For this review, take the finished solid that the model builds, in its own axes (mm). Face numbers are marked on the shaded views. A direction names the side the tool comes from. Round coordinates to 2 decimals unless told otherwise and drop trailing zeros. Loops run counter-clockwise (first coordinate to the right, second up) from the corner with the lowest first, then second, coordinate; pieces in that order, holes last.
1) Take a section at A-A (y = 2.25). State the section outline as (x, z) points.
2) Take a section at C-C (z = 1.75). State the section outline as (x, y) points, then the cut area to 3 significant figures.
3) Tool access review of the marked faces 4 and 5: name each direction out of +Z, -Z, +X, -X, +Y, -Y from which nothing blocks a thin tool from reaching the whole face with its end or side.
4) Wall thickness on L1, parallel to Z at x = -3.5, y = 5.25; L2, parallel to Y at x = 0.25, z = 1; L3, parallel to Y at x = 1.75, z = 1.5: over which ranges is each line inside the solid? List them lowest first.
5) Insertion check: pin 1 (1.5 mm diameter, centred on y = 5, z = 2, fed in from +X); pin 2 (1 mm diameter, centred on y = 6, z = 5, fed in from +X). Each pin has a flat end and moves straight along its axis. Give the tip position at first contact, or say it passes through.
6) Take a section at D-D (y = 1). State the section outline as (x, z) points, then the cut area to 3 significant figures.
7) Take a section at B-B (x = 2). State the section outline as (y, z) points.
8) Mouldability with a two-part tool opening along Z and no side actions: class the marked faces 1, 2 and 3 as pulls with the +Z half, pulls with the -Z half, needs draft (parallel to the pull), parting line crosses it, or undercut.
Autodesk Inventor part; units mm, degrees
ref_plane "作業平面1" through (-1.8159, 9, 6.1283) normal (0, 0.2337903, -0.972287) x (1, 0, 0)
ref_plane "YZ Plane" through (0, 0, 0) normal (1, 0, 0) x (0, 1, 0)
ref_plane "XZ Plane" through (0, 0, 0) normal (0, 1, 0) x (-1, 0, 0)
sketch "スケッチ1" plane through (0, 0, 0) normal (0, 0, 1) x (1, 0, 0)
  line L0 (-5, 9) -> (5, 9)
  line L1 (5, 9) -> (5, 0)
  line L2 (5, 0) -> (-5, 0)
  line L3 (-5, 0) -> (-5, 9)
  line L4 (-8.0749, 9) -> (-5, 9) construction
  point P0 (0, 0)
  point P1 (0, 9)
  point P2 (0, 0)
  dimension "d0" = 9
  dimension "d1" = 10
  dimension "d2" = 10
extrude "押し出し1" add sketch "スケッチ1" along normal blind 3
sketch "スケッチ2" plane through (-5, 9, 0) normal (0, 1, 0) x (1, 0, 0)
  line L0 (0, -3) -> (10, -3)
  line L1 (0, 0) -> (10, 0)
  line L2 (2.5173, -3) -> (0, 0)
  line L3 (10, 0) -> (7.4827, -3)
  line L4 (0, 0) -> (0, -3)
  line L5 (10, 0) -> (10, -3)
  point P0 (5, 0)
  dimension "d5" = 80
  dimension "d6" = 40
  dimension "d7" = 40
extrude "押し出し2" cut sketch "スケッチ2" against normal through all contours L4 L2 L0 | L3 L5 L0
sketch "スケッチ3" plane through (-5, 0, 0) normal (-0.7660444, 0, 0.6427876) x (0.6427876, 0, 0.7660444)
  line L0 (3.9162, 0) -> (0, 0)
  line L1 (3.9162, 9) -> (3.9162, 0)
  line L2 (0, 9) -> (3.9162, 9)
  line L3 (0, 9) -> (0, 0)
  line L4 (3.9162, 0) -> (7.1079, 0)
  line L5 (3.9162, 0) -> (-11.0838, 7)
  point P0 (3.2139, 0)
  point P1 (0, 1.8276)
  dimension "d10" = 15
  dimension "d11" = 7
extrude "押し出し3" cut sketch "スケッチ3" against normal through all contours L0 L3 L5
sketch "スケッチ4" plane through (5, 0, 0) normal (0.7660444, 0, 0.6427876) x (0.6427876, 0, -0.7660444)
  line L0 (0, 0) -> (-3.9162, 0)
  line L1 (0, 0) -> (0, 9)
  line L2 (-3.9162, 9) -> (0, 9)
  line L3 (-3.9162, 0) -> (-3.9162, 9)
  line L4 (-3.9162, 0) -> (11.0838, 7)
  point P0 (-3.2139, 0)
  point P1 (0, 1.8276)
  dimension "d14" = 15
  dimension "d15" = 7
extrude "押し出し4" cut sketch "スケッチ4" against normal through all contours L0 L4 L1
sketch "スケッチ5" plane through (0, 0, 3) normal (0, 0, 1) x (1, 0, 0)
  line L0 (-2.4827, 9) -> (-2.4827, 0)
  line L1 (-2.4827, 0) -> (2.4827, 0)
  line L2 (2.4827, 0) -> (2.4827, 9)
  line L3 (2.4827, 9) -> (-2.4827, 9)
  point P0 (0, 0)
extrude "押し出し5" add sketch "スケッチ5" along normal blind 10
sketch "スケッチ6" plane through (-2.4827, 0, 3) normal (-1, 0, 0) x (0, 0, 1)
  line L0 (0, 9) -> (0, 0)
  line L1 (0, 0) -> (10, 0)
  line L2 (10, 9) -> (10, 0)
  line L3 (0, 9) -> (10, 9)
  point P0 (-3, 0)
extrude "押し出し6" add sketch "スケッチ6" along normal blind 10
sketch "スケッチ7" plane through (2.4827, 0, 3) normal (1, 0, 0) x (0, 0, -1)
  line L0 (0, 0) -> (0, 9)
  line L1 (0, 9) -> (-10, 9)
  line L2 (-10, 0) -> (-10, 9)
  line L3 (0, 0) -> (-10, 0)
  point P0 (3, 0)
extrude "押し出し7" add sketch "スケッチ7" along normal blind 10
sketch "スケッチ8" plane through (5, 1.8276, 0) normal (0.7660444, 0, 0.6427876) x (0.6427876, 0, -0.7660444)
  line L0 (-7.1079, 7.1724) -> (-7.1079, -1.8276)
  line L1 (-3.9162, -1.8276) -> (0, 0)
  line L2 (0, 0) -> (0, 7.1724)
  line L3 (-3.9162, 7.1724) -> (0, 7.1724)
  line L4 (-3.9162, -1.8276) -> (-3.9162, 7.1724)
  line L5 (-3.9162, 20) -> (16.0838, 20)
  line L6 (16.0838, 20) -> (16.0838, -10)
  line L7 (16.0838, -10) -> (-3.9162, -10)
  line L8 (-3.9162, -10) -> (-3.9162, 20)
  point P0 (-3.2139, -1.8276)
  point P1 (-3.9162, -1.8276)
  point P2 (-3.9162, 7.1724)
extrude "押し出し8" cut sketch "スケッチ8" along normal through all
sketch "スケッチ9" plane through (-5, 1.8276, 0) normal (-0.7660444, 0, 0.6427876) x (0.6427876, 0, 0.7660444)
  line L0 (0, 0) -> (3.9162, -1.8276)
  line L1 (3.9162, 7.1724) -> (3.9162, -1.8276)
  line L2 (0, 7.1724) -> (3.9162, 7.1724)
  line L3 (0, 7.1724) -> (0, 0)
  line L4 (-16.0838, 20) -> (3.9162, 20)
  line L5 (3.9162, 20) -> (3.9162, -20)
  line L6 (3.9162, -20) -> (-16.0838, -20)
  line L7 (-16.0838, -20) -> (-16.0838, 20)
  point P0 (3.2139, -1.8276)
  point P1 (3.9162, 7.1724)
  point P2 (3.9162, -1.8276)
extrude "押し出し9" cut sketch "スケッチ9" along normal through all
sketch "スケッチ10" plane through (2.4827, 0, 3) normal (0.6427876, 0, -0.7660444) x (-0.7660444, 0, -0.6427876)
  line L0 (-13.0541, 9) -> (0, 9)
  line L1 (0, 0) -> (0, 9)
  line L2 (-1.5, 9) -> (0, 9)
  line L3 (0, 9) -> (0, 0)
  line L4 (0, 0) -> (-1.5, 0)
  line L5 (-1.5, 0) -> (-1.5, 9)
  line L6 (-13.0541, 9) -> (0, 9)
  line L7 (-13.0541, 0) -> (-13.0541, 9)
  line L8 (0, 0) -> (-13.0541, 0)
  line L9 (0, 0) -> (0, 9)
  line L10 (-20, 9) -> (-13.0541, 9)
  line L11 (-13.0541, 9) -> (-13.0541, 0)
  line L12 (-13.0541, 0) -> (-20, 0)
  line L13 (-20, 0) -> (-20, 9)
  line L14 (-13.0541, 0) -> (-13.0541, 9)
  line L15 (0, 0) -> (-13.0541, 0)
  point P0 (3.8302, 0)
  point P1 (-1.5, 0)
  dimension "d28" = 1.5
extrude "押し出し10" cut sketch "スケッチ10" against normal through all contours L0 L5 L8 L7 | L7 L12 L13 L10
sketch "スケッチ11" plane through (-2.4827, 0, 3) normal (-0.6427876, 0, -0.7660444) x (-0.7660444, 0, 0.6427876)
  line L0 (-7.6604, 9) -> (0, 9)
  line L1 (-4.0642, 0) -> (7.552, 0)
  line L2 (0, 9) -> (1.5, 9)
  line L3 (1.5, 9) -> (1.5, 0)
  line L4 (1.5, 0) -> (0, 0)
  line L5 (0, 0) -> (0, 9)
  line L6 (1.5, 9) -> (20, 9)
  line L7 (20, 9) -> (20, 0)
  line L8 (20, 0) -> (1.5, 0)
  line L9 (1.5, 0) -> (1.5, 9)
  line L10 (13.0541, 0) -> (0, 0)
  point P0 (-3.8302, 0)
  dimension "d31" = 1.5
extrude "押し出し11" cut sketch "スケッチ11" against normal through all contours L3 L6 L7 L8 L1
ref_plane "作業平面1" through (-1.8159, 9, 6.1283) normal (0, 0.2337903, -0.972287) x (1, 0, 0)
sketch "スケッチ12" plane through (-1.8159, 9, 6.1283) normal (0, 0.2337903, -0.972287) x (1, 0, 0)
  line L0 (-10, -6.5677) -> (20, -6.5677)
  line L1 (20, -6.5677) -> (20, 15.9547)
  line L2 (20, 15.9547) -> (-10, 15.9547)
  line L3 (-10, 15.9547) -> (-10, -6.5677)
  point P0 (1.8159, 10.1833)
extrude "押し出し12" cut sketch "スケッチ12" against normal through all
equation "\"d6\" = d7"
properties part number "antana_middle_ex"
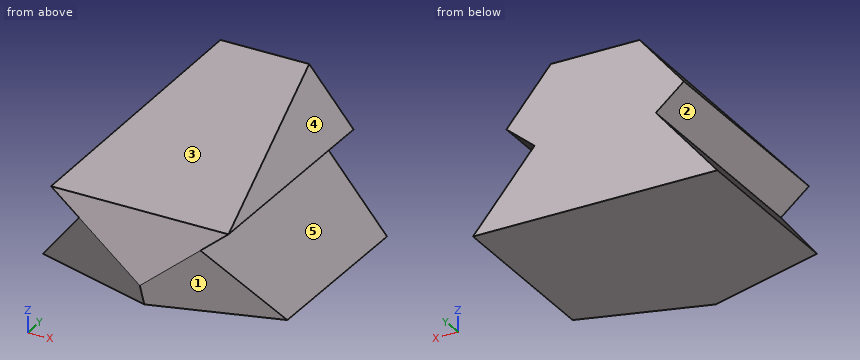
Response:
1. outline: (-5, 0) - (5, 0) - (2.48, 3) - (3.63, 3.96) - (3.18, 4.51) - (-3.18, 4.51) - (-3.63, 3.96) - (-2.48, 3) - close
2. outline: (-3.53, 0.76) - (-0.99, 0) - (0.99, 0) - (3.53, 0.76) - (3.53, 9) - (-3.53, 9) - close
2. area: 61.6 mm2
3. face 4: +Z, +X, +Y, -Y
3. face 5: +X, +Y, -Y
4. L1: z = 0 to 1.79, 3.85 to 4.12
4. L2: y = 0.05 to 9
4. L3: y = 0.32 to 9
5. pin 1: stops at x = 3.95
5. pin 2: stops at x = 3.18
6. outline: (-3.86, 1.36) - (-2.24, 0) - (2.24, 0) - (3.86, 1.36) - (2.48, 3) - (3.63, 3.96) - (3.43, 4.2) - (-3.43, 4.2) - (-3.63, 3.96) - (-2.48, 3) - close
6. area: 26.3 mm2
7. outline: (0, 2.59) - (0.93, 0) - (9, 0) - (9, 5.91) - (8.09, 5.91) - (0, 3.96) - close
8. face 1: pulls with the -Z half
8. face 2: undercut
8. face 3: pulls with the +Z half
